Here's how the part is built. I have some questions about the finished solid (model axes, mm). A direction names the side the tool comes from. Round coordinates to 2 decimals unless told otherwise and drop trailing zeros. Write each loop counter-clockwise with the first axis right and the second up, starting at its lowest first coordinate (ties: lowest second). Pieces come first, ordered by that corner, then holes. Notation, with made-up numbers: M 10.25,11 L 16.25,11 A27 ccw 16.25,43 Z; hole C -37,43 d4. An arc over 180 degrees is marked long. Write item = value, one per line. Start each with the question number.
(1) If we mould it in two halves opening along X, with no side actions, what happens to faces 6 (the flat face through (3, 101, 8)), 7 (the flat face through (99, 101, 0)), 8 (the flat face through (149.1, 99, 6))? For each: released by +X, released by -X, zero draft, split by the parting line, or undercut.
(2) On a 3-axis mill with a long thin cutter (end or side, diameter ignored), from which of +Z, -Z, +X, -X, +Y, -Y can I reach the whole of each face in a straight line? I mean faces 1 (the flat face through (192.71, 197, 7.06)), 2 (the flat face through (191, 194, 8)), 3 (the flat face through (192.6, 3, 8.8)), 4 (the flat face through (145, 99, 6)), 5 (the flat face through (43.597, 187, 9)). Say none if no direction works.
(3) I need wall thicknesses on line 1 along Y through (x, z) = (4.65, 8); line 2 along X through (y, z) = (185, 7.75); line 3 along X through (y, z) = (10.75, 8). Which ranges of each line are inside material? Lowest first, please.
(4) I want a section at A-A (x = 27). List the corners of the cut face in (y, z) for me.
(5) Will these pins go through, and if not, where does the flat tip stop? pin 1 Ø1.1 at (x, z) = (52, 7) entering from +Y; pin 2 Ø4.5 at (x, y) = (146.5, 65.5) entering from +Z; pin 3 Ø2.5 at (y, z) = (79.5, 7) entering from -X; pin 4 Ø3 at (x, z) = (76, 3) entering from -Y.
```python
from build123d import *

# Parameters (mm, degrees)
ESQUISSE1_W                 = 200
ESQUISSE1_H                 = 200
BOSS_EXTRU_PAROIE_DEPTH     = 4
BOSS_EXTRU_BORDS_DEPTH      = 8
BOSS_EXTRU_GLISSIERES_DEPTH = 5
CONG_1_R                    = 1
ESQUISSE8_W                 = 1.8
ESQUISSE8_H                 = 180
ENL_V_MAT_EXTRU_6_DEPTH     = 283.955826941
ESQUISSE5_R                 = 1.6
ENL_V_MAT_EXTRU_2_DEPTH     = 10
ENL_V_START                 = -10
ESQUISSE6_R                 = 1.6
ENL_V_MAT_EXTRU_3_DEPTH     = 10
ESQUISSE7_R                 = 1.6
ENL_V_MAT_EXTRU_4_DEPTH     = 10
ESQUISSE10_R                = 1.6
ENL_V_MAT_EXTRU_8_DEPTH     = 10
ESQUISSE11_W                = 113.303164178
ESQUISSE11_H                = 6
ENL_V_MAT_EXTRU_9_DEPTH     = 6
ESQUISSE9_R                 = 1.6
ENL_V_MAT_EXTRU_10_DEPTH    = 10


with BuildPart() as part:
    # Esquisse1 → Boss.-Extru. Paroie (new body)
    with BuildSketch(Plane.XY):
        with Locations((100, 100)):
            Rectangle(ESQUISSE1_W, ESQUISSE1_H)
    extrude(amount=BOSS_EXTRU_PAROIE_DEPTH)

    # Esquisse4 → Boss.-Extru. Bords (add)
    with BuildSketch(Plane.XY.offset(4)):
        Polygon((3, 3), (9, 3), (9, 184), (191, 184), (191, 3), (197, 3), (197, 197), (191, 197), (191, 190), (9, 190), (9, 197), (3, 197), align=None)
    extrude(amount=BOSS_EXTRU_BORDS_DEPTH)

    # Esquisse2 → Boss.-Extru. Glissieres (add)
    with BuildSketch(Plane.XY.offset(4)):
        with BuildLine():
            Line((47, 170), (53, 170))
            ThreePointArc((53, 170), (54.414213562, 169.414213562), (55, 168))
            Line((55, 168), (55, 32))
            ThreePointArc((55, 32), (54.414213562, 30.585786438), (53, 30))
            Line((53, 30), (47, 30))
            ThreePointArc((47, 30), (45.585786438, 30.585786438), (45, 32))
            Line((45, 32), (45, 168))
            ThreePointArc((45, 168), (45.585786438, 169.414213562), (47, 170))
        make_face()
        with BuildLine():
            Line((97, 170), (103, 170))
            ThreePointArc((103, 170), (104.414213562, 169.414213562), (105, 168))
            Line((105, 168), (105, 32))
            ThreePointArc((105, 32), (104.414213562, 30.585786438), (103, 30))
            Line((103, 30), (97, 30))
            ThreePointArc((97, 30), (95.585786438, 30.585786438), (95, 32))
            Line((95, 32), (95, 168))
            ThreePointArc((95, 168), (95.585786438, 169.414213562), (97, 170))
        make_face()
        with BuildLine():
            Line((147, 170), (153, 170))
            ThreePointArc((153, 170), (154.414213562, 169.414213562), (155, 168))
            Line((155, 168), (155, 32))
            ThreePointArc((155, 32), (154.414213562, 30.585786438), (153, 30))
            Line((153, 30), (147, 30))
            ThreePointArc((147, 30), (145.585786438, 30.585786438), (145, 32))
            Line((145, 32), (145, 168))
            ThreePointArc((145, 168), (145.585786438, 169.414213562), (147, 170))
        make_face()
    extrude(amount=BOSS_EXTRU_GLISSIERES_DEPTH)

    # Congé1
    cong_1_edges = [part.edges().sort_by_distance(p)[0] for p in [
        (200, 100, 4),
        (100, 200, 4),
        (0, 100, 4),
        (100, 0, 4),
    ]]
    fillet(cong_1_edges, radius=CONG_1_R)

    # Esquisse8 → Enlèv. mat.-Extru.6 (cut, through all)
    with BuildSketch(Plane.XY.offset(4)):
        with Locations((100, 85)):
            Rectangle(ESQUISSE8_W, ESQUISSE8_H)
        with Locations((150, 85)):
            Rectangle(ESQUISSE8_W, ESQUISSE8_H)
        with Locations((50, 85)):
            Rectangle(ESQUISSE8_W, ESQUISSE8_H)
    extrude(amount=ENL_V_MAT_EXTRU_6_DEPTH, mode=Mode.SUBTRACT)

    # Esquisse5 → Enlèv. mat.-Extru.2 (cut)
    with BuildSketch(Plane.ZY.offset(-3)):
        with Locations((8, 180)):
            Circle(ESQUISSE5_R)
        with Locations((8, 20)):
            Circle(ESQUISSE5_R)
    extrude(amount=-ENL_V_MAT_EXTRU_2_DEPTH, mode=Mode.SUBTRACT)

    # Esquisse6 → Enlèv. mat.-Extru.3 (cut)
    with BuildSketch(Plane(origin=(197, 0, 0), x_dir=(0, 0, -1), z_dir=(1, 0, 0)).offset(ENL_V_START)):
        with Locations(Location((-8, 180, 0), (0, 0, 180))):
            Circle(ESQUISSE6_R)
        with Locations(Location((-8, 20, 0), (0, 0, 180))):
            Circle(ESQUISSE6_R)
    extrude(amount=ENL_V_MAT_EXTRU_3_DEPTH, mode=Mode.SUBTRACT)

    # Esquisse7 → Enlèv. mat.-Extru.4 (cut)
    with BuildSketch(Plane.XZ.offset(-184)):
        with Locations(Location((35, 8, 0), (0, 0, 270))):
            Circle(ESQUISSE7_R)
        with Locations(Location((165, 8, 0), (0, 0, 270))):
            Circle(ESQUISSE7_R)
    extrude(amount=-ENL_V_MAT_EXTRU_4_DEPTH, mode=Mode.SUBTRACT)

    # Esquisse10 → Enlèv. mat.-Extru.8 (cut)
    with BuildSketch(Plane(origin=(0, 3, 0), x_dir=(-1, 0, 0), z_dir=(0, -1, 0))):
        with Locations(Location((-194.2, -8, 0), (0, 0, 90))):
            Circle(ESQUISSE10_R)
        with Locations(Location((-5.8, -8, 0), (0, 0, 90))):
            Circle(ESQUISSE10_R)
    extrude(amount=-ENL_V_MAT_EXTRU_8_DEPTH, mode=Mode.SUBTRACT)

    # Esquisse11 → Enlèv. mat.-Extru.9 (cut)
    with BuildSketch(Plane.XY.offset(12)):
        with Locations((100.248809194, 187)):
            Rectangle(ESQUISSE11_W, ESQUISSE11_H)
    extrude(amount=-ENL_V_MAT_EXTRU_9_DEPTH, mode=Mode.SUBTRACT)

    # Esquisse9 → Enlèv. mat.-Extru.10 (cut)
    with BuildSketch(Plane(origin=(0, 197, 0), x_dir=(1, 0, 0), z_dir=(0, 1, 0)).offset(ENL_V_START)):
        with Locations(Location((194.2, -8, 0), (0, 0, 90))):
            Circle(ESQUISSE9_R)
        with Locations(Location((5.8, -8, 0), (0, 0, 90))):
            Circle(ESQUISSE9_R)
    extrude(amount=ENL_V_MAT_EXTRU_10_DEPTH, mode=Mode.SUBTRACT)


solid = part.part
```
Returned:
q1.face_6 = released by -X
q1.face_7 = zero draft
q1.face_8 = undercut
q2.face_1 = +Z, +X, -X, +Y
q2.face_2 = +Z, +Y
q2.face_3 = +Z, +X, -X, -Y
q2.face_4 = +Z, -Y
q2.face_5 = +Z, +Y, -Y
q3.line_1 = 13 to 18.4, 21.6 to 178.4, 181.6 to 187
q3.line_2 = 3 to 33.42, 36.58 to 43.6, 156.9 to 163.42, 166.58 to 197
q3.line_3 = 3 to 4.2, 7.4 to 9, 191 to 192.6, 195.8 to 197
q4.outline = M 0,0 L 200,0 L 200,3 A1 ccw 199,4 L 190,4 L 190,12 L 184,12 L 184,4 L 1,4 A1 ccw 0,3 Z
q5.pin_1 = 170
q5.pin_2 = 9
q5.pin_3 = 3
q5.pin_4 = 0
